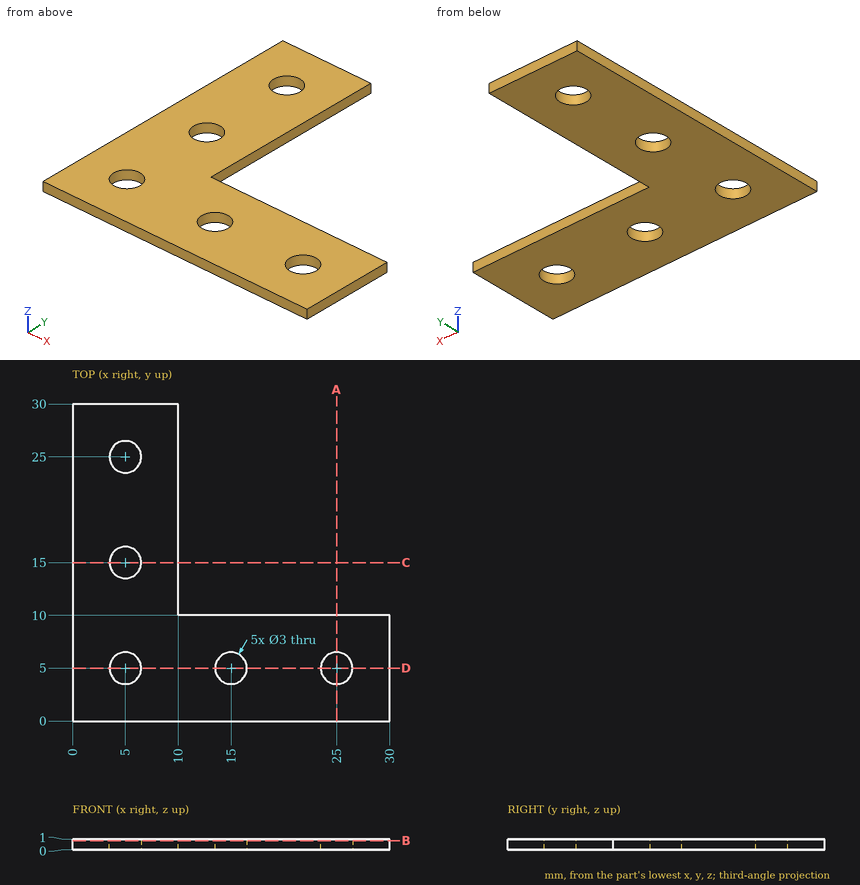
Source: three-view drawing plus pictorial views. Frame: mm from the lowest corner of the part. Give positions to 0.01 mm unless a question says otherwise; leave off trailing zeros. Order: outer loops, then holes, each group sorted by start corner. A loop starts at its lowest first (then second) coordinate and runs counter-clockwise, first axis right, second up. Notation, with made-up numbers: M 36,79.25 L 74,79.25 A31 cw 74,105.25 Z; hole C 5,32.5 d9. An arc over 180 degrees is marked long. Return JSON: item names as keys, results as strings.
Item 1: First-contact query: P1, Ø1.5, axis at x = 10.5, y = 26.5, coming from the +Z side. Flat tip, straight axial feed; report the tip coordinate or a pass-through.
Solutions:
{"P1": "z = 1"}
Item 2: Cut plane A-A (x = 25). Return loops of the section in (y, z).
Solutions:
{"outline": "M 0,0 L 3.5,0 L 3.5,1 L 0,1 Z; M 6.5,0 L 10,0 L 10,1 L 6.5,1 Z"}
Item 3: Cut plane B-B (z = 0.85). Return loops of the section in (x, y).
Solutions:
{"outline": "M 0,0 L 30,0 L 30,10 L 10,10 L 10,30 L 0,30 Z; hole C 5,5 d3; hole C 5,15 d3; hole C 5,25 d3; hole C 15,5 d3; hole C 25,5 d3"}
Item 4: Cut plane D-D (y = 5). Return loops of the section in (x, z), then the cut area to 3 significant figures.
Solutions:
{"outline": "M 0,0 L 3.5,0 L 3.5,1 L 0,1 Z; M 6.5,0 L 13.5,0 L 13.5,1 L 6.5,1 Z; M 16.5,0 L 23.5,0 L 23.5,1 L 16.5,1 Z; M 26.5,0 L 30,0 L 30,1 L 26.5,1 Z", "area": "21.0 mm^2"}
Item 5: Ray query, probe 1 along Y at (x, z) = (5, 0.35); probe 2 along Y at (x, z) = (25, 0.15); probe 3 along Y at (x, z) = (6, 0.7). Return the intervals inside material, ascending.
Solutions:
{"probe 1": "0 to 3.5, 6.5 to 13.5, 16.5 to 23.5, 26.5 to 30", "probe 2": "0 to 3.5, 6.5 to 10", "probe 3": "0 to 3.88, 6.12 to 13.88, 16.12 to 23.88, 26.12 to 30"}
